Geometry check sheet. Reference: drawing and pictorial views, mm from the part's lowest x, y, z. Round coordinates to 2 decimals unless told otherwise and drop trailing zeros. Order: outer loops, then holes, each group sorted by start corner. A loop starts at its lowest first (then second) coordinate and runs counter-clockwise, first axis right, second up.
(1) Cross-section at B-B on x = 6. Enter the section's corners in (y, z), and give its area (3 significant figures).
(2) Cross-section at A-A on z = 16.25. Enter the section's corners in (x, y), and give its area (3 significant figures).
(3) Cross-section at D-D on y = 9. Enter the section's corners in (x, z), and give its area (3 significant figures).
(4) Gauge pin test, flat ends, axial feed: P1, Ø3, axis at x = 57.5, y = 2, coming from the -Z side; P2, Ø6, axis at x = 66.5, y = 3.5, coming from the -Z side; P3, Ø3, axis at x = 29, y = 7, coming from the -Z side. Record the tip position at first contact, or that the pin passes through.
(5) Cross-section at C-C on y = 5. Enter the section's corners in (x, z), and give its area (3 significant figures).
(6) Thickness scan on L1, parallel to Y at x = 94, z = 9; L2, parallel to X at y = 7.25, z = 1; L3, parallel to X at y = 7.5, z = 7.25. Record the ranges inside material, lowest first.
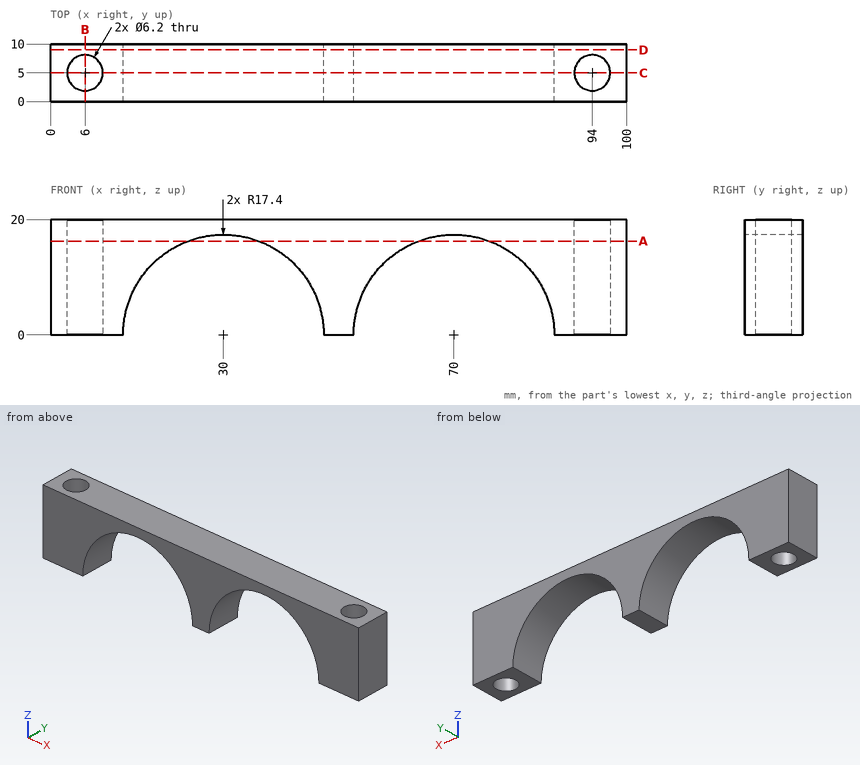
Found:
1. outline: (0, 0) - (1.9, 0) - (1.9, 20) - (0, 20) - close; (8.1, 0) - (10, 0) - (10, 20) - (8.1, 20) - close
1. area: 76.0 mm2
2. outline: (0, 0) - (23.78, 0) - (23.78, 10) - (0, 10) - close; (36.22, 0) - (63.78, 0) - (63.78, 10) - (36.22, 10) - close; (76.22, 0) - (100, 0) - (100, 10) - (76.22, 10) - close; hole circle Ø6.2 at (6, 5); hole circle Ø6.2 at (94, 5)
2. area: 691 mm2
3. outline: (0, 0) - (12.6, 0) arc R17.4 cw to (47.4, 0) - (52.6, 0) arc R17.4 cw to (87.4, 0) - (100, 0) - (100, 20) - (0, 20) - close
3. area: 1,050 mm2
4. P1: stops at z = 10.33
4. P2: stops at z = 16.14
4. P3: stops at z = 17.22
5. outline: (0, 0) - (2.9, 0) - (2.9, 20) - (0, 20) - close; (9.1, 0) - (12.6, 0) arc R17.4 cw to (47.4, 0) - (52.6, 0) arc R17.4 cw to (87.4, 0) - (90.9, 0) - (90.9, 20) - (9.1, 20) - close; (97.1, 0) - (100, 0) - (100, 20) - (97.1, 20) - close
5. area: 801 mm2
6. L1: y = 0 to 1.9, 8.1 to 10
6. L2: x = 0 to 3.87, 8.13 to 12.63, 47.37 to 52.63, 87.37 to 91.87, 96.13 to 100
6. L3: x = 0 to 4.17, 7.83 to 14.18, 45.82 to 54.18, 85.82 to 92.17, 95.83 to 100
